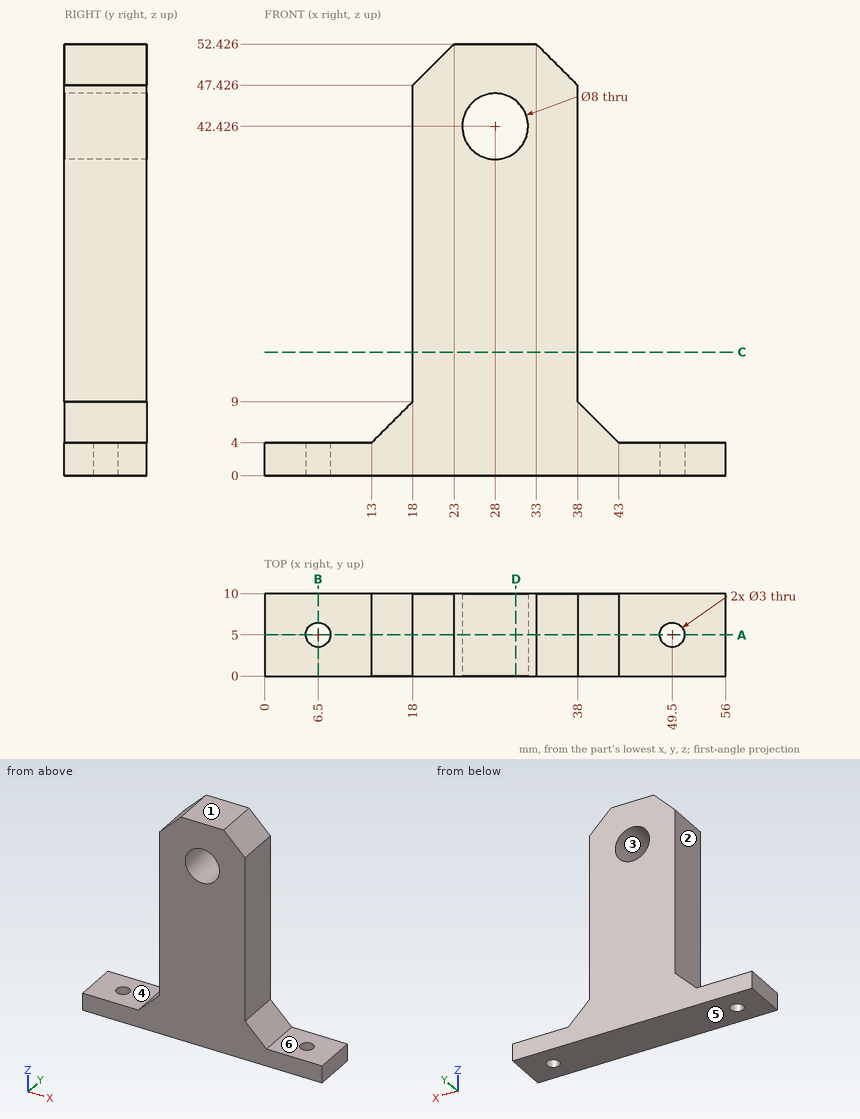
Here's the drawing with two shaded views (mm, measured from the low corner). I have some questions. A direction names the side the tool comes from. Give positions to 0.01 mm unless a question says otherwise; leave off trailing zeros. Write each loop counter-clockwise with the first axis right and the second up, starting at its lowest first coordinate (ties: lowest second). Pieces come first, ordered by that corner, then holes. Notation, with made-up numbers: (-35, 60) -> (-30, 60) arc R19 cw to (-30, 96) -> close; hole circle Ø7 at (13.25, -15.5). An arc over 180 degrees is marked (long way). One line per item, written item: value.
Q1. We'd pull the mould along X, two halves only. Please class the marked faces 1, 2 and 3: +X half, -X half, draft (parallel to the pull), parting line (faces both ways), or undercut.
Results found:
face 1: draft
face 2: -X half
face 3: undercut
Q2. Imagine slicing it at A-A on y = 5. Please give me the cut outline in (x, z), and give its area (3 significant figures).
Results found:
outline: (0, 0) -> (5, 0) -> (5, 4) -> (0, 4) -> close; (8, 0) -> (48, 0) -> (48, 4) -> (43, 4) -> (38, 9) -> (38, 47.43) -> (33, 52.43) -> (23, 52.43) -> (18, 47.43) -> (18, 9) -> (13, 4) -> (8, 4) -> close; (51, 0) -> (56, 0) -> (56, 4) -> (51, 4) -> close; hole circle Ø8 at (28, 42.43)
area: 1,120 mm^2
Q3. Imagine slicing it at B-B on x = 6.5. Please give me the cut outline in (y, z).
Results found:
outline: (0, 0) -> (3.5, 0) -> (3.5, 4) -> (0, 4) -> close; (6.5, 0) -> (10, 0) -> (10, 4) -> (6.5, 4) -> close
Q4. Which directions (+Z, -Z, +X, -X, +Y, -Y) give clear straight access to the entire face, cutting with the end or side of a thin tool? Please do the marked faces 4, 5 and 6.
Results found:
face 4: +Z, -X, +Y, -Y
face 5: -Z, +X, -X, +Y, -Y
face 6: +Z, +X, +Y, -Y
Q5. Please list where these lines run through material, in increasing order: line 1 (X direction, y = 5, z = 3.1); line 2 (Z direction, x = 28, y = 2.75); line 3 (Y direction, x = 6.5, z = 1.7). Write a range as [from, to].
Results found:
line 1: x = [0, 5], [8, 48], [51, 56]
line 2: z = [0, 38.43], [46.43, 52.43]
line 3: y = [0, 3.5], [6.5, 10]
Q6. Imagine slicing it at C-C on z = 15. Please give me the cut outline in (x, y), and give its area (3 significant figures).
Results found:
outline: (18, 0) -> (38, 0) -> (38, 10) -> (18, 10) -> close
area: 200 mm^2
Q7. For P1, Ø5, axis at y = 7, z = 37.5, coming from the +X side; P2, Ø3, axis at x = 12, y = 8.5, coming from the +Z side; P3, Ø4, axis at x = 42.5, y = 2.5, coming from the +Z side; P4, Ø1.5, axis at x = 39.5, z = 39.5, coming from the +Y side, each with a flat end and sliding along its axis, tell me the tip position at first contact or that it passes through.
Results found:
P1: stops at x = 38
P2: stops at z = 4.5
P3: stops at z = 6.5
P4: passes through
Q8. Imagine slicing it at D-D on x = 30.5. Please give me the cut outline in (y, z), and give its area (3 significant figures).
Results found:
outline: (0, 0) -> (10, 0) -> (10, 39.3) -> (0, 39.3) -> close; (0, 45.55) -> (10, 45.55) -> (10, 52.43) -> (0, 52.43) -> close
area: 462 mm^2
